Work out the finished part from the listing and answer in its coordinate system (mm). Face numbers are marked on the shaded views. A direction names the side the tool comes from. Give positions to 0.01 mm unless a question says otherwise; leave off trailing zeros. Write each loop counter-clockwise with the first axis right and the second up, starting at its lowest first coordinate (ties: lowest second). Pieces come first, ordered by that corner, then holes. Notation, with made-up numbers: (67.25, 81) -> (93.25, 81) arc R30 cw to (93.25, 109) -> close; hole circle Ø6 at (41, -30). An arc over 180 degrees is marked (long way). Use a Markdown table: item, result. Add a question column.
Q1. Section A-A, the plane x = 0 is taken. Give the vertices of the cut face in (y, z), plus the area to 3 significant figures.
Q2. Section B-B, the plane y = -20.5 is taken. Give the vertices of the cut face in (x, z).
Q3. Consider line 1 (Y direction, x = 8, z = 22); line 2 (X direction, y = -18.5, z = 11.5); line 3 (Y direction, x = -21.5, z = 9.75). Determine where each line is inside the solid, lowest interval first.
Q4. Each of these flat-tipped pins is pushed along its axis until it touches: pin 1 Ø1 at (y, z) = (7, 12) entering from +X; pin 2 Ø4 at (x, z) = (-19, 18) entering from +Y; pin 3 Ø1 at (y, z) = (-6, 11.5) entering from -X. Where does it stop, or does it pass through?
Q5. For the marked faces 1, 2 and 3, determine the directions among +Z, -Z, +X, -X, +Y, -Y from which every point of the face is accessible in a straight line to the end or side of a thin tool.
Q6. For a pull along Y with two mould halves and no side action, classify the marked faces 4, 5 and 6 as pulls with the +Y half, pulls with the -Y half, needs draft (parallel to the pull), parting line crosses it, or undercut.
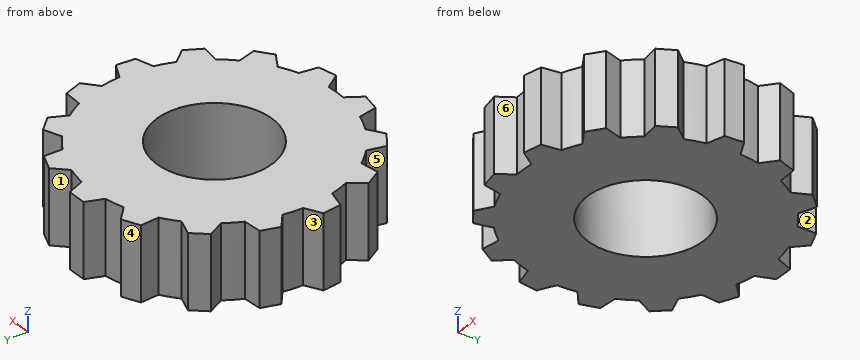
from build123d import *

# Parameters (mm, degrees)
BOSS_EXTRUDE1_DEPTH = 30
SKETCH2_R           = 23.45019305
CUT_EXTRUDE1_DEPTH  = 30


with BuildPart() as part:
    # Sketch1 → Boss-Extrude1 (new body)
    with BuildSketch(Plane.XY):
        with BuildLine():
            Line((6.50170184, 49.57547653), (3.772289399, 56.49452457))
            Line((3.772289399, 56.49452457), (-3.772289399, 56.49452457))
            Line((-3.772289399, 56.49452457), (-6.50170184, 49.57547653))
            ThreePointArc((-6.50170184, 49.57547653), (-10.395584541, 48.907380037), (-14.22456272, 47.933931775))
            Line((-14.22456272, 47.933931775), (-19.532235431, 53.144644629))
            Line((-19.532235431, 53.144644629), (-26.424551121, 50.075987976))
            Line((-26.424551121, 50.075987976), (-26.103763086, 42.644971014))
            ThreePointArc((-26.103763086, 42.644971014), (-29.389262615, 40.450849719), (-32.491271159, 38.00417475))
            Line((-32.491271159, 38.00417475), (-39.459459309, 40.605572828))
            Line((-39.459459309, 40.605572828), (-44.507767895, 34.998858134))
            Line((-44.507767895, 34.998858134), (-41.192246548, 28.340762592))
            ThreePointArc((-41.192246548, 28.340762592), (-43.301270189, 25), (-45.139943641, 21.503150654))
            Line((-45.139943641, 21.503150654), (-52.563784195, 21.045428595))
            Line((-52.563784195, 21.045428595), (-54.895187259, 13.870107767))
            Line((-54.895187259, 13.870107767), (-49.158216363, 9.13617885))
            ThreePointArc((-49.158216363, 9.13617885), (-49.726094768, 5.226423163), (-49.983509784, 1.28403646))
            Line((-49.983509784, 1.28403646), (-56.579353267, -2.153661434))
            Line((-56.579353267, -2.153661434), (-55.790730039, -9.656910239))
            Line((-55.790730039, -9.656910239), (-48.624283981, -11.648133214))
            ThreePointArc((-48.624283981, -11.648133214), (-47.552825815, -15.450849719), (-46.184473, -19.157099304))
            Line((-46.184473, -19.157099304), (-50.811838152, -24.980363835))
            Line((-50.811838152, -24.980363835), (-47.039548753, -31.514160735))
            Line((-47.039548753, -31.514160735), (-39.68277116, -30.418377226))
            ThreePointArc((-39.68277116, -30.418377226), (-37.157241274, -33.456530318), (-34.399721261, -36.285798561))
            Line((-34.399721261, -36.285798561), (-36.258494609, -43.48773439))
            Line((-36.258494609, -43.48773439), (-30.154802146, -47.922326542))
            Line((-30.154802146, -47.922326542), (-23.879746699, -43.929007473))
            ThreePointArc((-23.879746699, -43.929007473), (-20.336832154, -45.677272882), (-16.666945204, -47.1403536))
            Line((-16.666945204, -47.1403536), (-15.43572795, -54.475680595))
            Line((-15.43572795, -54.475680595), (-8.0560163, -56.04428673))
            Line((-8.0560163, -56.04428673), (-3.947697093, -49.843913246))
            ThreePointArc((-3.947697093, -49.843913246), (0, -50), (3.947697093, -49.843913246))
            Line((3.947697093, -49.843913246), (8.056016301, -56.04428673))
            Line((8.056016301, -56.04428673), (15.43572795, -54.475680595))
            Line((15.43572795, -54.475680595), (16.666945204, -47.1403536))
            ThreePointArc((16.666945204, -47.1403536), (20.336832154, -45.677272882), (23.879746699, -43.929007473))
            Line((23.879746699, -43.929007473), (30.154802146, -47.922326542))
            Line((30.154802146, -47.922326542), (36.258494609, -43.48773439))
            Line((36.258494609, -43.48773439), (34.399721261, -36.285798561))
            ThreePointArc((34.399721261, -36.285798561), (37.157241274, -33.456530318), (39.68277116, -30.418377226))
            Line((39.68277116, -30.418377226), (47.039548753, -31.514160735))
            Line((47.039548753, -31.514160735), (50.811838152, -24.980363835))
            Line((50.811838152, -24.980363835), (46.184473, -19.157099304))
            ThreePointArc((46.184473, -19.157099304), (47.552825815, -15.450849719), (48.624283981, -11.648133214))
            Line((48.624283981, -11.648133214), (55.790730039, -9.656910239))
            Line((55.790730039, -9.656910239), (56.579353267, -2.153661433))
            Line((56.579353267, -2.153661433), (49.983509784, 1.28403646))
            ThreePointArc((49.983509784, 1.28403646), (49.726094768, 5.226423163), (49.158216363, 9.13617885))
            Line((49.158216363, 9.13617885), (54.895187259, 13.870107767))
            Line((54.895187259, 13.870107767), (52.563784195, 21.045428595))
            Line((52.563784195, 21.045428595), (45.139943641, 21.503150654))
            ThreePointArc((45.139943641, 21.503150654), (43.301270189, 25), (41.192246548, 28.340762592))
            Line((41.192246548, 28.340762592), (44.507767895, 34.998858134))
            Line((44.507767895, 34.998858134), (39.459459309, 40.605572828))
            Line((39.459459309, 40.605572828), (32.491271159, 38.00417475))
            ThreePointArc((32.491271159, 38.00417475), (29.389262615, 40.450849719), (26.103763086, 42.644971014))
            Line((26.103763086, 42.644971014), (26.424551121, 50.075987976))
            Line((26.424551121, 50.075987976), (19.53223543, 53.144644629))
            Line((19.53223543, 53.144644629), (14.22456272, 47.933931775))
            ThreePointArc((14.22456272, 47.933931775), (10.395584541, 48.907380037), (6.50170184, 49.57547653))
        make_face()
    extrude(amount=BOSS_EXTRUDE1_DEPTH)

    # Sketch2 → Cut-Extrude1 (cut)
    with BuildSketch(Plane.XY.offset(30)):
        Circle(SKETCH2_R)
    extrude(amount=-CUT_EXTRUDE1_DEPTH, mode=Mode.SUBTRACT)


solid = part.part
Result set:
| question | item | result |
|---|---|---|
| 1 | outline | (-50, 0) -> (-23.45, 0) -> (-23.45, 30) -> (-50, 30) -> close; (23.45, 0) -> (56.49, 0) -> (56.49, 30) -> (23.45, 30) -> close |
| 1 | area | 1,790 mm2 |
| 2 | outline | (-47.25, 0) -> (-11.39, 0) -> (-11.39, 30) -> (-47.25, 30) -> close; (11.39, 0) -> (47.25, 0) -> (47.25, 30) -> (11.39, 30) -> close |
| 3 | line 1 | y = -55.96 to -22.04, 22.04 to 49.36 |
| 3 | line 2 | x = -46.45 to -14.41, 14.41 to 46.45 |
| 3 | line 3 | y = -45.14 to -9.36, 9.36 to 52.27 |
| 4 | pin 1 | stops at x = 49.58 |
| 4 | pin 2 | stops at y = 53.14 |
| 4 | pin 3 | stops at x = -56.23 |
| 5 | face 1 | +Z, -Z, +Y |
| 5 | face 2 | +Z, -Z, +X |
| 5 | face 3 | +Z, -Z, -X |
| 6 | face 4 | pulls with the +Y half |
| 6 | face 5 | undercut |
| 6 | face 6 | pulls with the -Y half |
